Geometry check sheet. Reference: the model listing, model coordinates, mm. A direction names the side the tool comes from. Round coordinates to 2 decimals unless told otherwise and drop trailing zeros. Write each loop counter-clockwise with the first axis right and the second up, starting at its lowest first coordinate (ties: lowest second). Pieces come first, ordered by that corner, then holes.
Autodesk Fusion 360 part; units mm, degrees
sketch "Skizze1" plane through (0, 0, 0) normal (0, 1, 0) x (1, 0, 0)
  circle A0 centre (0, 0) radius 10
  circle A1 centre (0, 0) radius 15
  circle A2 centre (50, 0) radius 7.5
  line L0 (2.25, 14.8303) -> (51.125, 7.4151)
  line L1 (51.125, -7.4151) -> (2.25, -14.8303)
  dimension "d1" = 20
  dimension "d2" = 5
  dimension "d3" = 15
  dimension "d5" = 50
extrude "Extrusion1" add sketch "Skizze1" along normal mid plane 5
sketch "Skizze2" plane through (0, 0, 0) normal (0, 0, 1) x (1, 0, 0)
  line L0 (2.25, 2.5) -> (2.25, -2.5)
  line L1 (2.25, -2.5) -> (51.125, -2.5)
sketch "Skizze3" plane through (0, 0, 0) normal (0, 0, 1) x (1, 0, 0)
  line L0 (17.5, 2.5) -> (57.5, 2.5)
  line L1 (57.5, 2.5) -> (57.5, 1)
  line L2 (57.5, 1) -> (51.1276, 2.5)
  line L3 (51.1276, 2.5) -> (50.7745, 1)
  line L4 (50.7745, 1) -> (44.4021, 2.5)
  line L5 (44.4021, 2.5) -> (44.049, 1)
  line L6 (44.049, 1) -> (37.6765, 2.5)
  line L7 (37.6765, 2.5) -> (37.3235, 1)
  line L8 (37.3235, 1) -> (30.951, 2.5)
  line L9 (30.951, 2.5) -> (30.5979, 1)
  line L10 (30.5979, 1) -> (24.2255, 2.5)
  line L11 (24.2255, 2.5) -> (23.8724, 1)
  line L12 (23.8724, 1) -> (17.5, 2.5)
  line L13 (23.8724, 1) -> (57.5, 1) construction
  line L14 (24.2255, 2.5) -> (51.1276, 2.5) construction
  line L15 (51.125, -2.5) -> (51.125, 2.5)
  line L16 (2.25, 2.5) -> (51.125, 2.5)
  line L17 (1.75, 0) -> (22.5, 0)
  line L18 (44.049, -1) -> (37.6765, -2.5)
  line L19 (23.8724, -1) -> (17.5, -2.5)
  line L20 (17.5, -2.5) -> (57.5, -2.5)
  line L21 (24.2255, -2.5) -> (23.8724, -1)
  line L22 (30.951, -2.5) -> (30.5979, -1)
  line L23 (51.1276, -2.5) -> (50.7745, -1)
  line L24 (37.3235, -1) -> (30.951, -2.5)
  line L25 (23.8724, -1) -> (57.5, -1) construction
  line L26 (24.2255, -2.5) -> (51.1276, -2.5) construction
  line L27 (57.5, -2.5) -> (57.5, -1)
  line L28 (37.6765, -2.5) -> (37.3235, -1)
  line L29 (57.5, -1) -> (51.1276, -2.5)
  line L30 (50.7745, -1) -> (44.4021, -2.5)
  line L31 (44.4021, -2.5) -> (44.049, -1)
  line L32 (30.5979, -1) -> (24.2255, -2.5)
  line L33 (51.125, -2.5) -> (51.125, 2.5)
  line L34 (57.5, 2.5) -> (51.125, 2.5)
  line L35 (51.125, 2.5) -> (51.125, -2.5)
  line L36 (51.125, -2.5) -> (57.5, -2.5)
  point P0 (51.125, -2.5)
  dimension "d10" = 40
  dimension "d11" = 1.5
extrude "Extrusion2" cut sketch "Skizze3" along normal mid plane 30 contours L0 L1 L2 L34 | L20 L27 L29 L36 | L19 L20 L21 | L20 L22 L32 | L20 L24 L28 | L18 L20 L31 | L15 L20 L23 L30 L33 L35 | L0 L3 L4 L15 L16 L33 L35 | L0 L5 L6 L16 | L0 L7 L8 L16 | L0 L9 L10 L16 | L0 L11 L12 L16
fillet "Abrundung1" radius 2 2 edges at (-9.3233, 2.5, -3.6162) (-9.3233, -2.5, 3.6162)
fillet "Abrundung2" radius 1 6 edges at (9.875, 2.5, -13.6735) (-15, 2.5, 0) (9.875, 2.5, 13.6735) (9.875, -2.5, 13.6735) (-15, -2.5, 0) (9.875, -2.5, -13.6735)
1. Depth check by flat-ended pin: pin 1 Ø10 at (x, z) = (7, 7.5) entering from +Y; pin 2 Ø3 at (y, z) = (0, 2.5) entering from -X; pin 3 Ø6 at (x, z) = (6, -6.5) entering from -Y. Enter the tip coordinate at first touch or a pass-through.
2. Scan lines: line 1 along Z through (x, y) = (0, 0.1); line 2 along X through (y, z) = (-0.15, 0); line 3 along Z through (x, y) = (-5, 0.9). Record each from-to range of solid material in increasing order.
3. Section check A-A (x = 0). Record the cut outline in (y, z), plus the area to 3 significant figures.
4. Access from +Z, -Z, +X, -X, +Y, -Y to the whole of each face (thin tool, end or side, straight path). Record for faces 1 (the face through (50.953, -1.76, -0.105)), 2 (the face through (9.924, -2.215, -13.362)), 3 (the face through (20.73, 1.74, -0.17)).
5. Section check B-B (x = 40). Record the cut outline in (y, z).
6. Section check C-C (x = 49). Record the cut outline in (y, z).
Results below:
1. pin 1: stops at y = 2.5
1. pin 2: stops at x = -14.97
1. pin 3: stops at y = -2.49
2. line 1: z = -15 to -10, 10 to 15
2. line 2: x = -15 to -10, 10 to 57.5
2. line 3: z = -14.14 to -8.71, 8.71 to 14.14
3. outline: (-2.5, -14) arc R1 ccw to (-1.5, -15) - (1.5, -15) arc R1 ccw to (2.5, -14) - (2.5, -12) arc R2 ccw to (0.5, -10) - (-0.5, -10) arc R2 ccw to (-2.5, -12) - close; (-2.5, 12) arc R2 ccw to (-0.5, 10) - (0.5, 10) arc R2 ccw to (2.5, 12) - (2.5, 14) arc R1 ccw to (1.5, 15) - (-1.5, 15) arc R1 ccw to (-2.5, 14) - close
3. area: 45.7 mm2
4. face 1: +Z, -Z, -Y
4. face 2: -Z, +X, -Y
4. face 3: +Z, -Z, +Y
5. outline: (-1.95, -9.1) - (1.95, -9.1) - (1.95, 9.1) - (-1.95, 9.1) - close
6. outline: (-1.42, -7.74) - (1.42, -7.74) - (1.42, 7.74) - (-1.42, 7.74) - close
